```python
from build123d import *

# Parameters (mm, degrees)
SKETCH1_W           = 53.4573
SKETCH1_H           = 13
SKETCH1_R           = 4.2
BOSS_EXTRUDE1_DEPTH = 50.3
BOSS_EXTRUDE2_START = -15
SKETCH3_R           = 4.2
BOSS_EXTRUDE2_DEPTH = 15
SKETCH8_W           = 15.5
SKETCH8_H           = 13
BOSS_EXTRUDE3_DEPTH = 10.6
CHAMFER1_SIZE       = 10.6
SKETCH5_R           = 3
SKETCH5_R_2         = 4
CUT_EXTRUDE1_DEPTH  = 76.366988286
CUT_EXTRUDE2_DEPTH  = 5.3
BOSS_EXTRUDE4_DEPTH = 10
CUT_EXTRUDE3_DEPTH  = 1
SKETCH13_W          = 21.695080859
SKETCH13_H          = 9.09610943
CUT_EXTRUDE4_DEPTH  = 3
SKETCH16_R          = 1.65
CUT_EXTRUDE5_DEPTH  = 59.425257644
SKETCH17_R          = 7.3
CUT_EXTRUDE6_DEPTH  = 10.5
SKETCH15_W          = 4
SKETCH15_H          = 8
CUT_EXTRUDE7_DEPTH  = 60.472016368
SKETCH18_R          = 8.3
CUT_EXTRUDE8_DEPTH  = 1.2
SKETCH21_R          = 1.65
CUT_EXTRUDE9_DEPTH  = 60.472016368
CUT_EXTRUDE10_DEPTH = 2.6
FILLET1_R           = 2
CUT_EXTRUDE11_START = -1
CUT_EXTRUDE11_DEPTH = 10


# Read off the part's stored shape, not the designer's step: Cut-Extrude11
with BuildPart() as part:
    # Sketch1 → Boss-Extrude1 (new body)
    with BuildSketch(Plane.XY):
        Rectangle(SKETCH1_W, SKETCH1_H)
        with Locations(Location((-20, 0, 0), (0, 0, 180))):
            Circle(SKETCH1_R, mode=Mode.SUBTRACT)
        with Locations(Location((20, 0, 0), (0, 0, 180))):
            Circle(SKETCH1_R, mode=Mode.SUBTRACT)
    extrude(amount=BOSS_EXTRUDE1_DEPTH)

    # Sketch3 → Boss-Extrude2 (add)
    with BuildSketch(Plane.XY.offset(50.3).offset(BOSS_EXTRUDE2_START)):
        with Locations(Location((-20, 0, 0), (0, 0, 180))):
            Circle(SKETCH3_R)
        with Locations(Location((20, 0, 0), (0, 0, 180))):
            Circle(SKETCH3_R)
    extrude(amount=BOSS_EXTRUDE2_DEPTH)

    # Sketch8 → Boss-Extrude3 (add)
    with BuildSketch(Plane(origin=(0, 6.5, 0), x_dir=(1, 0, 0), z_dir=(0, 1, 0))):
        with Locations((0, -6.5)):
            Rectangle(SKETCH8_W, SKETCH8_H)
    extrude(amount=BOSS_EXTRUDE3_DEPTH)

    # Chamfer1
    chamfer1_edges = [part.edges().sort_by_distance(p)[0] for p in [
        (7.75, 6.5, 6.5),
        (-7.75, 6.5, 6.5),
    ]]
    chamfer(chamfer1_edges, length=CHAMFER1_SIZE - 0.0001)  # a hair under: the kernel refuses the full size

    # Sketch5 → Cut-Extrude1 (cut, through all)
    with BuildSketch(Plane.ZY.offset(26.72865)):
        with Locations(Location((6.5, 12.5, 0), (0, 0, 270))):
            Circle(SKETCH5_R)
        with Locations((36.5, 12.5)):
            Circle(SKETCH5_R_2)
    extrude(amount=-CUT_EXTRUDE1_DEPTH, mode=Mode.SUBTRACT)

    # Sketch10 → Cut-Extrude2 (cut)
    with BuildSketch(Plane.ZY):
        Polygon((2.516283143, 14.8), (2.516283143, 17.1), (10.483716857, 17.1), (10.483716857, 14.8), (10.483716857, 10.2), (6.5, 7.9), (2.516283143, 10.2), align=None)
    cut_extrude2 = extrude(amount=-CUT_EXTRUDE2_DEPTH, mode=Mode.SUBTRACT)

    # Mirror1: Cut-Extrude2 across plane
    add(cut_extrude2.mirror(Plane.ZY), mode=Mode.SUBTRACT)

    # Sketch11 → Boss-Extrude4 (add)
    with BuildSketch(Plane.ZY.offset(26.72865)):
        with BuildLine():
            Line((33.035176772, 15.964823228), (29.509293572, 15.964823228))
            Line((29.509293572, 15.964823228), (22.7, 6.5))
            Line((22.7, 6.5), (50.3, 6.5))
            Line((50.3, 6.5), (43.490706428, 15.964823228))
            Line((43.490706428, 15.964823228), (39.964823228, 15.964823228))
            ThreePointArc((39.964823228, 15.964823228), (36.5, 7.6), (33.035176772, 15.964823228))
        make_face()
    boss_extrude4 = extrude(amount=-BOSS_EXTRUDE4_DEPTH)

    # Sketch12 → Cut-Extrude3 (cut)
    with BuildSketch(Plane.ZY.offset(24.72865)):
        with BuildLine():
            Line((30.15, 12.5), (30.15, 21.960655534))
            Line((30.15, 21.960655534), (42.85, 21.960655534))
            Line((42.85, 21.960655534), (42.85, 12.5))
            ThreePointArc((42.85, 12.5), (36.5, 6.15), (30.15, 12.5))
        make_face()
    cut_extrude3 = extrude(amount=-CUT_EXTRUDE3_DEPTH, mode=Mode.SUBTRACT)

    # Sketch13 → Cut-Extrude4 (cut)
    with BuildSketch(Plane.ZY.offset(26.72865)):
        with Locations((35.453328021, 17.048054715)):
            Rectangle(SKETCH13_W, SKETCH13_H)
    cut_extrude4 = extrude(amount=-CUT_EXTRUDE4_DEPTH, mode=Mode.SUBTRACT)

    # Mirror2: Boss-Extrude4, Cut-Extrude3, Cut-Extrude4 across plane
    add(boss_extrude4.mirror(Plane.ZY))
    add(cut_extrude3.mirror(Plane.ZY), mode=Mode.SUBTRACT)
    add(cut_extrude4.mirror(Plane.ZY), mode=Mode.SUBTRACT)

    # Sketch16 → Cut-Extrude5 (cut, through all)
    with BuildSketch(Plane(origin=(0, 6.5, 0), x_dir=(1, 0, 0), z_dir=(0, 1, 0))):
        with Locations(Location((0, -29.3, 0), (0, 0, 180))):
            Circle(SKETCH16_R)
    extrude(amount=-CUT_EXTRUDE5_DEPTH, mode=Mode.SUBTRACT)

    # Sketch17 → Cut-Extrude6 (cut)
    with BuildSketch(Plane(origin=(0, 6.5, 0), x_dir=(1, 0, 0), z_dir=(0, 1, 0))):
        with Locations(Location((0, -29.3, 0), (0, 0, 180))):
            Circle(SKETCH17_R)
    extrude(amount=-CUT_EXTRUDE6_DEPTH, mode=Mode.SUBTRACT)

    # Sketch15 → Cut-Extrude7 (cut, through all)
    with BuildSketch(Plane(origin=(0, 0, 0), x_dir=(-1, 0, 0), z_dir=(0, 0, -1))):
        with Locations((-5.3, 0)):
            Rectangle(SKETCH15_W, SKETCH15_H)
    cut_extrude7 = extrude(amount=-CUT_EXTRUDE7_DEPTH, mode=Mode.SUBTRACT)

    # Mirror3: Cut-Extrude7 across plane
    add(cut_extrude7.mirror(Plane.ZY), mode=Mode.SUBTRACT)

    # Sketch18 → Cut-Extrude8 (cut)
    with BuildSketch(Plane(origin=(0, 6.5, 0), x_dir=(1, 0, 0), z_dir=(0, 1, 0))):
        with Locations(Location((0, -29.3, 0), (0, 0, 180))):
            Circle(SKETCH18_R)
    extrude(amount=-CUT_EXTRUDE8_DEPTH, mode=Mode.SUBTRACT)

    # Sketch20 → Revolve1 (revolve)
    with BuildSketch(Plane.ZY, mode=Mode.PRIVATE) as revolve1_sk:
        Polygon((30.95, -4), (30.95, -2), (31.95, -2), (33.95, -4), align=None)
    revolve(revolve1_sk.sketch.rotate(Axis((0, -4, 29.3), (0, 1, 0)), 270), axis=Axis((0, -4, 29.3), (0, 1, 0)))

    # Sketch21 → Cut-Extrude9 (cut, through all)
    with BuildSketch(Plane.XY.offset(50.3)):
        with Locations((20, 0)):
            Circle(SKETCH21_R)
        with Locations((-20, 0)):
            Circle(SKETCH21_R)
    extrude(amount=-CUT_EXTRUDE9_DEPTH, mode=Mode.SUBTRACT)

    # Sketch22 → Cut-Extrude10 (cut)
    with BuildSketch(Plane.XY.offset(46.3)):
        Polygon((-22.814582562, 1.414434516), (-22.814582562, 2.989434516), (-17.185417438, 2.989434516), (-17.185417438, 1.497865113), (-17.185417438, -1.625), (-17.185417438, -7.227237341), (-22.814582562, -7.227237341), (-22.814582562, -1.625), align=None)
    cut_extrude10 = extrude(amount=-CUT_EXTRUDE10_DEPTH, mode=Mode.SUBTRACT)

    # Mirror4: Cut-Extrude10 across plane
    add(cut_extrude10.mirror(Plane.ZY), mode=Mode.SUBTRACT)

    # Fillet1
    fillet1_edges = [part.edges().sort_by_distance(p)[0] for p in [
        (26.72865, 0, 0),
        (26.72865, 0, 50.3),
        (-26.72865, 0, 0),
        (-26.72865, 0, 50.3),
    ]]
    fillet(fillet1_edges, radius=FILLET1_R)

    # Cut-Extrude11 outline → Cut-Extrude11 (cut)
    with BuildSketch(Plane(origin=(0, -4, 0), x_dir=(1, 0, 0), z_dir=(0, 1, 0)).offset(CUT_EXTRUDE11_START)):
        with BuildLine():
            ThreePointArc((3.3, -20.391577019), (5.485502581, -21.543759839), (7.3, -23.220526339))
            Line((7.3, -23.220526339), (7.3, -2))
            Line((7.3, -2), (3.3, -2))
            Line((3.3, -2), (3.3, -20.391577019))
        make_face()
        with BuildLine():
            Line((-7.3, -2), (-7.3, -23.220526339))
            ThreePointArc((-7.3, -23.220526339), (-5.485502581, -21.543759839), (-3.3, -20.391577019))
            Line((-3.3, -20.391577019), (-3.3, -2))
            Line((-3.3, -2), (-7.3, -2))
        make_face()
    extrude(amount=CUT_EXTRUDE11_DEPTH, mode=Mode.SUBTRACT)


solid = part.part
```
Can you work these out from the model? Positions are in its coordinate system, mm. A direction names the side the tool comes from. Round coordinates to 2 decimals unless told otherwise and drop trailing zeros. Loops run counter-clockwise (first coordinate to the right, second up) from the corner with the lowest first, then second, coordinate; pieces in that order, holes last.
Item 1: If we mould it in two halves opening along Y, with no side actions, what happens to faces 1 (the flat face through (0, 0, 50.3)), 2 (the flat face through (-3.3, 0, 43)), 3 (the flat face through (21.799, 11.299, 26.152))? For each: +Y half, -Y half, draft (parallel to the pull), parting line (faces both ways), or undercut.
Item 2: Suppose I cut it at A-A, the plane x = -20. Write out the boundary of the cut face in (y, z), then the cut area to 3 significant figures.
Item 3: Please list where these lines run through material, in increasing order: L1, parallel to Y at x = -20, z = 49; L2, parallel to Y at x = 20, z = 7.5; L3, parallel to X at y = 12.75, z = 42.
Item 4: Will these pins go through, and if not, where does the flat tip stop? pin 1 Ø1.1 at (x, z) = (19.5, 31) entering from +Y; pin 2 Ø4.5 at (x, y) = (20, 0) entering from -Z; pin 3 Ø15 at (x, z) = (-7.5, 31) entering from +Y.
Item 5: Which directions (+Z, -Z, +X, -X, +Y, -Y) give clear straight access to the entire face, cutting with the end or side of a thin tool? Please do faces 4 (the flat face through (23.729, 7, 36)), 5 (the flat face through (25, 12.5, 44)), 6 (the flat face through (6, 4, 23)).
Item 6: Suppose I cut it at C-C, the plane z = 7.5. State how many separate pieces and enclosed holes the cut face has, then the cut area to 3 significant figures.
Item 7: Suppose I cut it at B-B, the plane z = 15. Write out the boundary of the cut face in (x, y), then the cut area to 3 significant figures.
Reported:
1. face 1: draft
1. face 2: undercut
1. face 3: +Y half
2. outline: (-6.5, 0) - (-4.2, 0) - (-4.2, 35.3) - (-1.65, 35.3) - (-1.65, 43.7) - (-6.5, 43.7) - close; (-6.5, 46.3) - (-1.65, 46.3) - (-1.65, 50.3) - (-6.5, 50.3) - close; (1.65, 35.3) - (4.2, 35.3) - (4.2, 0) - (6.5, 0) - (6.5, 22.7) - (15.96, 29.51) - (15.96, 33.04) arc R4.9 cw (long way) to (15.96, 39.96) - (15.96, 43.49) - (6.5, 50.3) - (1.65, 50.3) - (1.65, 46.3) - (2.99, 46.3) - (2.99, 43.7) - (1.65, 43.7) - close
2. area: 420 mm2
3. L1: y = -6.5 to -1.65, 1.65 to 8.31
3. L2: y = -6.5 to -4.2, 4.2 to 6.5
3. L3: x = -23.73 to -16.73, 16.73 to 23.73
4. pin 1: stops at y = 15.96
4. pin 2: stops at z = 35.3
4. pin 3: stops at y = 6.5
5. face 4: +Y
5. face 5: +Z, -Z, +X, +Y
5. face 6: +Z, -Z
6. separate pieces: 3
6. enclosed holes: 4
6. area: 610 mm2
7. outline: (-26.73, -6.5) - (26.73, -6.5) - (26.73, 6.5) - (-26.73, 6.5) - close; hole circle Ø8.4 at (-20, 0); hole (-7.3, -5) - (-3.3, -5) - (-3.3, 5) - (-7.3, 5) - close; hole (3.3, -5) - (7.3, -5) - (7.3, 5) - (3.3, 5) - close; hole circle Ø8.4 at (20, 0)
7. area: 504 mm2
